Can you work these out from the drawing? Everything is in mm from the part's minimum corner. A direction names the side the tool comes from. Round coordinates to 2 decimals unless told otherwise and drop trailing zeros. Loops run counter-clockwise (first coordinate to the right, second up) from the corner with the lowest first, then second, coordinate; pieces in that order, holes last. Notation, with made-up numbers: M -2,37 L 54,37 A24 ccw 54,48 Z; hole C 85.25,50 d3. An arc over 180 degrees is marked long. Use a Markdown table: item, result.
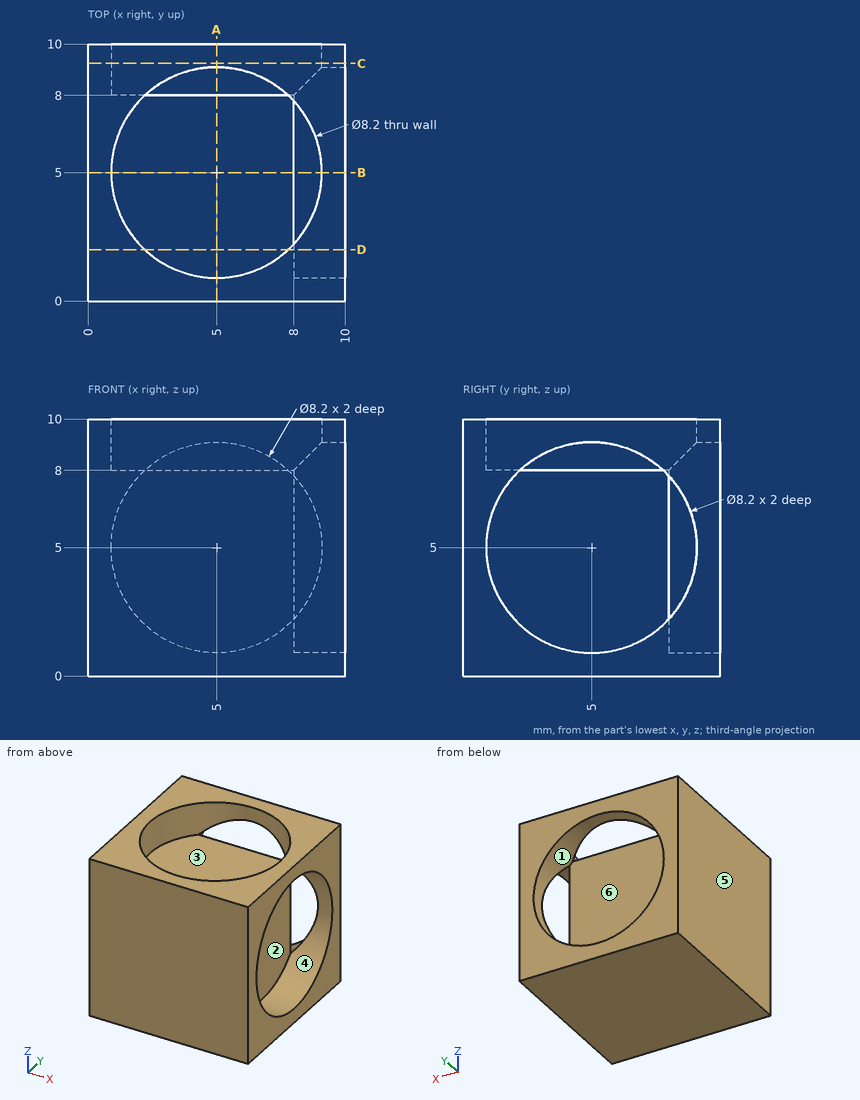
Q1. Will these pins go through, and if not, where does the flat tip stop? P1, Ø5.5, axis at y = 5, z = 5, coming from the +X side; P2, Ø2, axis at x = 5, z = 6, coming from the +Y side; P3, Ø5, axis at x = 4, y = 4.5, coming from the +Z side.
Return value:
| item | result |
|---|---|
| P1 | stops at x = 8 |
| P2 | stops at y = 8 |
| P3 | stops at z = 8 |
Q2. For the marked faces 1, 2 and 3, which set-ups out of +Z, -Z, +X, -X, +Y, -Y let a thin tool reach every point of the face, with its end or its side?
Return value:
| item | result |
|---|---|
| face 1 | +Y |
| face 2 | +X |
| face 3 | +Z |
Q3. Imagine slicing it at A-A, the plane x = 5. Please give me the cut outline in (y, z).
Return value:
| item | result |
|---|---|
| outline | M 0,0 L 10,0 L 10,0.9 L 8,0.9 L 8,8 L 0.9,8 L 0.9,10 L 0,10 Z; M 9.1,9.1 L 10,9.1 L 10,10 L 9.1,10 Z |
Q4. I need wall thicknesses on line 1 (X direction, y = 5, z = 9.5); line 2 (X direction, y = 8.8, z = 5). Which ranges of each line are inside material? Lowest first, please. Write a range as from..to.
Return value:
| item | result |
|---|---|
| line 1 | x = 0..0.9, 9.1..10 |
| line 2 | x = 0..0.9 |
Q5. We'd pull the mould along Y, two halves only. Please class the marked faces 4, 5 and 6: pulls with the +Y half, pulls with the -Y half, needs draft (parallel to the pull), parting line crosses it, or undercut.
Return value:
| item | result |
|---|---|
| face 4 | undercut |
| face 5 | needs draft |
| face 6 | pulls with the +Y half |
Q6. Imagine slicing it at C-C, the plane y = 9.25. Please give me the cut outline in (x, z).
Return value:
| item | result |
|---|---|
| outline | M 0,0 L 10,0 L 10,10 L 0,10 Z; hole C 5,5 d8.2 |
Q7. Imagine slicing it at D-D, the plane y = 2. Please give me the cut outline in (x, z), then the cut area to 3 significant figures.
Return value:
| item | result |
|---|---|
| outline | M 0,0 L 10,0 L 10,2.21 L 8,2.21 L 8,7.79 L 10,7.79 L 10,10 L 7.79,10 L 7.79,8 L 2.21,8 L 2.21,10 L 0,10 Z |
| area | 77.6 mm^2 |
